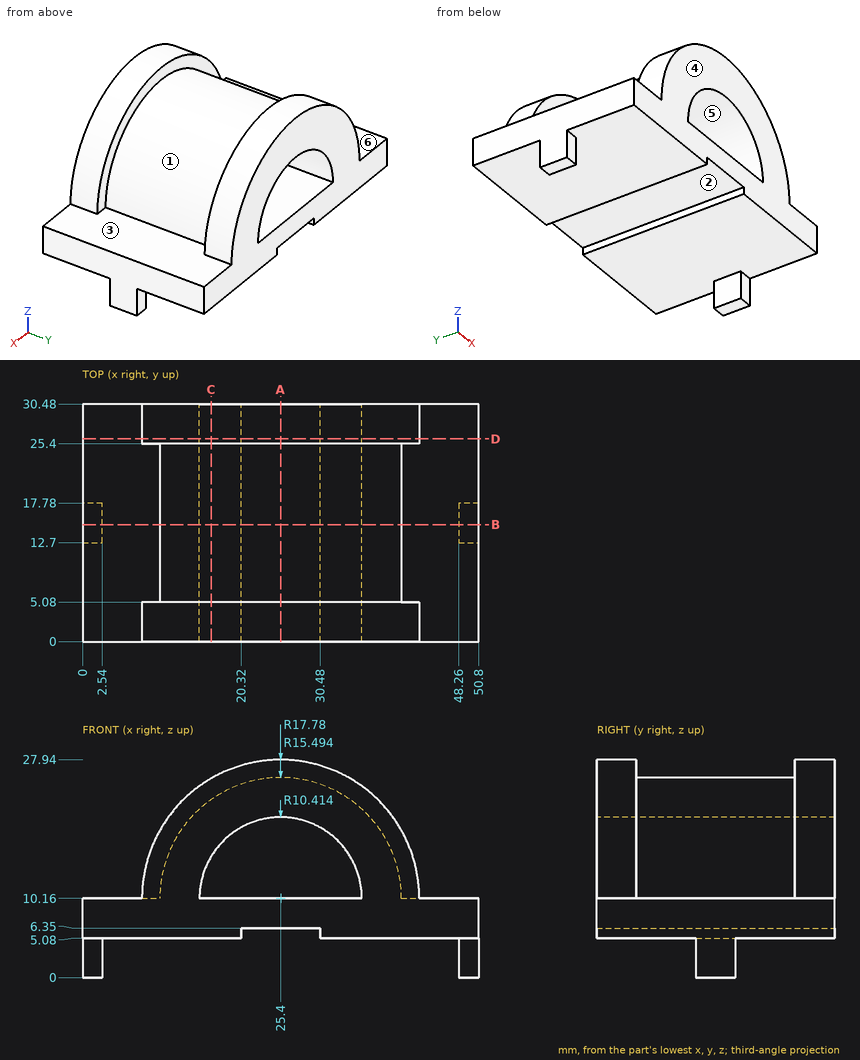
Source: three-view drawing plus pictorial views. Frame: mm from the lowest corner of the part. A direction names the side the tool comes from. Round coordinates to 2 decimals unless told otherwise and drop trailing zeros. Write each loop counter-clockwise with the first axis right and the second up, starting at its lowest first coordinate (ties: lowest second). Pieces come first, ordered by that corner, then holes. Notation, with made-up numbers: M 85.25,66 L 107.25,66 A14 cw 107.25,80 Z; hole C 83,82 d9. An arc over 180 degrees is marked long. Write each question's results on one line, items separated by ' | '.
Q1. Line query: line 1 along Y through (x, z) = (10.5, 19); line 2 along Z through (x, y) = (5, 23.5); line 3 along Z through (x, y) = (23, 19). Output: solid intervals per line, ascending.
Results:
line 1: y = 0 to 5.08, 25.4 to 30.48 | line 2: z = 5.08 to 10.16 | line 3: z = 6.35 to 10.16, 20.29 to 25.47
Q2. Draft query along Z for the marked faces 4, 5 and 6. Return one class per face: released by +Z, released by -Z, zero draft, split by the parting line, or undercut.
Results:
face 4: zero draft | face 5: undercut | face 6: released by +Z
Q3. Access query for the marked faces 1, 2 and 3. Directions: +Z, -Z, +X, -X, +Y, -Y. A direction counts if a zero-diameter tool reaches every point of the face in a straight line with its end or side. Return the directions, or none.
Results:
face 1: +Z | face 2: -Z, +Y, -Y | face 3: +Z, +X
Q4. Section query C-C (x = 16.5). Return loops of the section in (y, z).
Results:
outline: M 0,5.08 L 30.48,5.08 L 30.48,10.16 L 0,10.16 Z; M 0,15.57 L 30.48,15.57 L 30.48,25.55 L 25.4,25.55 L 25.4,22.84 L 5.08,22.84 L 5.08,25.55 L 0,25.55 Z
Q5. Section query D-D (y = 26). Return loops of the section in (x, z), and give its area (3 significant figures).
Results:
outline: M 0,5.08 L 20.32,5.08 L 20.32,6.35 L 30.48,6.35 L 30.48,5.08 L 50.8,5.08 L 50.8,10.16 L 43.18,10.16 A17.78 ccw 7.62,10.16 L 0,10.16 Z; hole M 14.99,10.16 L 35.81,10.16 A10.41 ccw Z | area: 571 mm^2
Q6. Section query B-B (y = 15). Return loops of the section in (x, z).
Results:
outline: M 0,0 L 2.54,0 L 2.54,5.08 L 20.32,5.08 L 20.32,6.35 L 30.48,6.35 L 30.48,5.08 L 48.26,5.08 L 48.26,0 L 50.8,0 L 50.8,10.16 L 40.89,10.16 A15.49 ccw 9.91,10.16 L 0,10.16 Z; hole M 14.99,10.16 L 35.81,10.16 A10.41 ccw Z
Q7. Pin query (flat end, axial travel): P1, Ø10.5, axis at x = 24.5, y = 19, coming from the +Z side; P2, Ø6, axis at y = 27.5, z = 24, coming from the -X side; P3, Ø11, axis at x = 26, y = 12, coming from the -Z side. Return the tip coordinate at first contact, or that it passes through.
Results:
P1: stops at z = 25.65 | P2: stops at x = 11.31 | P3: stops at z = 5.08
Q8. Section query A-A (x = 25.4). Return loops of the section in (y, z), and give its area (3 significant figures).
Results:
outline: M 0,6.35 L 30.48,6.35 L 30.48,10.16 L 0,10.16 Z; M 0,20.57 L 30.48,20.57 L 30.48,27.94 L 25.4,27.94 L 25.4,25.65 L 5.08,25.65 L 5.08,27.94 L 0,27.94 Z | area: 294 mm^2
